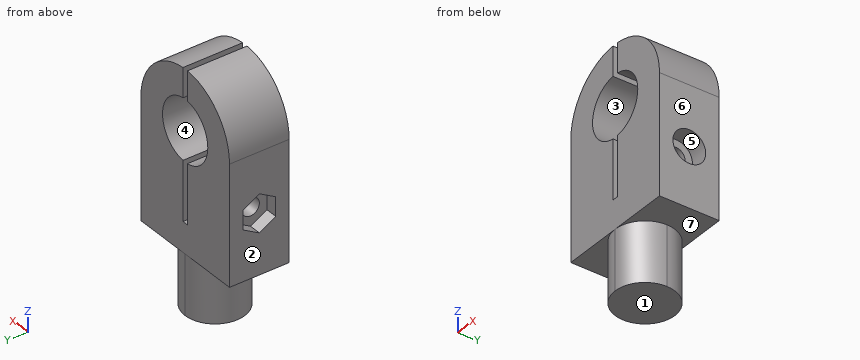
from build123d import *

# Parameters (mm, degrees)
F0_R      = 5.1
F1_DEPTH  = 10
F2_R      = 1.5
F3_DEPTH  = 25
F5_DEPTH  = 25
F7_DEPTH  = 10
F8_R      = 2.75
F8_R_2    = 1.5
F9_DEPTH  = 3
F10_R     = 1.5
F11_DEPTH = 2


with BuildPart() as f1:
    # F0 (on Front) → F1 (new body)
    with BuildSketch(Plane.XZ):
        with BuildLine():
            ThreePointArc((-10, 0), (0, -10), (10, 0))
            ThreePointArc((10, 0), (0, 10), (-10, 0))
        make_face()
        Circle(F0_R, mode=Mode.SUBTRACT)
        with BuildLine():
            Line((10, -20), (10, 0))
            ThreePointArc((10, 0), (0, -10), (-10, 0))
            Line((-10, 0), (-10, -20))
            Line((-10, -20), (10, -20))
        make_face()
    extrude(amount=F1_DEPTH)

    # F2 (on face) → F3 (cut)
    with BuildSketch(Plane(origin=(-10, 0, 0), x_dir=(0, -1, 0), z_dir=(-1, 0, 0))):
        with Locations((5, -10)):
            Circle(F2_R)
    extrude(amount=-F3_DEPTH, mode=Mode.SUBTRACT)

    # F4 (on face) → F5 (cut)
    with BuildSketch(Plane.XZ.offset(10)):
        with BuildLine():
            Line((0.5, 12.5812012702), (-0.5, 12.5812012702))
            Line((-0.5, 12.5812012702), (-0.5, 9.9874921777))
            ThreePointArc((-0.5, 9.9874921777), (0, 10), (0.5, 9.9874921777))
            Line((0.5, 9.9874921777), (0.5, 12.5812012702))
        make_face()
        with BuildLine():
            ThreePointArc((0.5, 9.9874921777), (0, 10), (-0.5, 9.9874921777))
            Line((-0.5, 9.9874921777), (-0.5, 5.0754310162))
            ThreePointArc((-0.5, 5.0754310162), (0, 5.1), (0.5, 5.0754310162))
            Line((0.5, 5.0754310162), (0.5, 9.9874921777))
        make_face()
        with BuildLine():
            ThreePointArc((0.5, -5.0754310162), (0, -5.1), (-0.5, -5.0754310162))
            Line((-0.5, -5.0754310162), (-0.5, -15))
            Line((-0.5, -15), (0.5, -15))
            Line((0.5, -15), (0.5, -5.0754310162))
        make_face()
        with BuildLine():
            ThreePointArc((0.5, 5.0754310162), (0, 5.1), (-0.5, 5.0754310162))
            Line((-0.5, 5.0754310162), (-0.5, -5.0754310162))
            ThreePointArc((-0.5, -5.0754310162), (0, -5.1), (0.5, -5.0754310162))
            Line((0.5, -5.0754310162), (0.5, 5.0754310162))
        make_face()
    extrude(amount=-F5_DEPTH, mode=Mode.SUBTRACT)

    # F6 (on face) → F7 (join)
    with BuildSketch(Plane(origin=(0, 0, -20), x_dir=(1, 0, 0), z_dir=(0, 0, -1))):
        with BuildLine():
            ThreePointArc((0, 0), (3.5355339059, 1.4644660941), (5, 5))
            ThreePointArc((5, 5), (3.5355339059, 8.5355339059), (0, 10))
            ThreePointArc((0, 10), (-5, 5), (0, 0))
        make_face()
    extrude(amount=F7_DEPTH)

    # F8 (on face) → F9 (cut)
    with BuildSketch(Plane.YZ.offset(10)):
        with Locations((-5, -10)):
            Circle(F8_R)
        with Locations((-5, -10)):
            Circle(F8_R_2, mode=Mode.SUBTRACT)
    extrude(amount=-F9_DEPTH, mode=Mode.SUBTRACT)

    # F10 (on face) → F11 (cut)
    with BuildSketch(Plane(origin=(-10, 0, 0), x_dir=(0, -1, 0), z_dir=(-1, 0, 0))):
        Polygon((7.75, -11.5877132403), (7.75, -8.4122867597), (5, -6.8245735195), (2.25, -8.4122867597), (2.25, -11.5877132403), (5, -13.1754264805), align=None)
        with Locations((5, -10)):
            Circle(F10_R, mode=Mode.SUBTRACT)
    extrude(amount=-F11_DEPTH, mode=Mode.SUBTRACT)


solid = f1.part
Could you check a few things on this model? Use its own coordinates, in mm. Face numbers are marked on the shaded views. A direction names the side the tool comes from. Give positions to 0.01 mm unless a question says otherwise; leave off trailing zeros. Order: outer loops, then holes, each group sorted by start corner. A loop starts at its lowest first (then second) coordinate and runs counter-clockwise, first axis right, second up. Notation, with made-up numbers: (84, -8.5) -> (109, -8.5) arc R11 ccw to (109, -1.5) -> close; hole circle Ø8 at (58, -7). An arc over 180 degrees is marked (long way). Return JSON: item names as keys, results as strings.
1. On a 3-axis mill with a long thin cutter (end or side, diameter ignored), from which of +Z, -Z, +X, -X, +Y, -Y can I reach the whole of each face in a straight line? I mean the marked faces 5, 6 and 7. Say none if no direction works.
Answer list:
{"face 5": "+X", "face 6": "+Z, -Z, +X, +Y, -Y", "face 7": "-Z, +X"}
2. Thinking about a two-plate mould opening in X: for the marked faces 1, 2, 3 and 4, which applies, pulls with the +X half, pulls with the -X half, needs draft (parallel to the pull), parting line crosses it, or undercut?
Answer list:
{"face 1": "needs draft", "face 2": "pulls with the -X half", "face 3": "undercut", "face 4": "undercut"}
3. Imagine slicing it at C-C on y = -5.5. Give the number of separate pieces and of enclosed holes in the cut face, then the cut area to 3 significant figures.
Answer list:
{"separate pieces": "3", "enclosed holes": "0", "area": "493 mm2"}
4. Imagine slicing it at B-B on z = -10. List the corners of the cut face in (x, y) for me, then the cut area to 4 significant figures.
Answer list:
{"outline": "(-10, -10) -> (-0.5, -10) -> (-0.5, -6.5) -> (-8, -6.5) -> (-8, -7.75) -> (-10, -7.75) -> close; (-10, -2.25) -> (-8, -2.25) -> (-8, -3.5) -> (-0.5, -3.5) -> (-0.5, 0) -> (-10, 0) -> close; (0.5, -10) -> (10, -10) -> (10, -7.75) -> (7, -7.75) -> (7, -6.5) -> (0.5, -6.5) -> close; (0.5, -3.5) -> (7, -3.5) -> (7, -2.25) -> (10, -2.25) -> (10, 0) -> (0.5, 0) -> close", "area": "120.5 mm2"}
5. Imagine slicing it at D-D on x = 7.5. List the corners of the cut face in (y, z) for me.
Answer list:
{"outline": "(-10, -20) -> (0, -20) -> (0, 6.61) -> (-10, 6.61) -> close; hole circle Ø5.5 at (-5, -10)"}
6. For pin 1 Ø1.5 at (x, z) = (-7, -21) entering from +Y; pin 2 Ø4 at (y, z) = (-3, 2.5) entering from +X; pin 3 Ø1.5 at (y, z) = (-5.5, 7) entering from +X; pin 4 Ø1.5 at (y, z) = (-3, 8.5) entering from -X, each with a flat end and sliding along its axis, tell me the tip position at first contact or that it passes through.
Answer list:
{"pin 1": "passes through", "pin 2": "stops at x = 9.99", "pin 3": "stops at x = 7.81", "pin 4": "stops at x = -6.32"}
7. Imagine slicing it at A-A on z = -5.5. List the corners of the cut face in (x, y) for me.
Answer list:
{"outline": "(-10, -10) -> (-0.5, -10) -> (-0.5, 0) -> (-10, 0) -> close; (0.5, -10) -> (10, -10) -> (10, 0) -> (0.5, 0) -> close"}
8. I need wall thicknesses on line 1 (X direction, y = -0.5, z = -11); line 2 (Z direction, x = -4, y = -5); line 3 (Y direction, x = 4.25, z = -10). Which ranges of each line are inside material? Lowest first, please. Write a range as from..to.
Answer list:
{"line 1": "x = -10..-0.5, 0.5..10", "line 2": "z = -30..-11.5, -8.5..-3.16, 3.16..9.17", "line 3": "y = -10..-6.5, -3.5..0"}
